Here's how the part is built. I have some questions about the finished solid (model axes, mm). Give positions to 0.01 mm unless a question says otherwise; leave off trailing zeros. Write each loop counter-clockwise with the first axis right and the second up, starting at its lowest first coordinate (ties: lowest second). Pieces come first, ordered by that corner, then holes. Notation, with made-up numbers: (51.25, 29) -> (79.25, 29) arc R24 ccw to (79.25, 41) -> close; hole circle Ø9 at (38.25, 40.25). An arc over 180 degrees is marked (long way). Use one line per item in the form item = value.
```python
from build123d import *

# Parameters (mm, degrees)
TUBE_SQUARE_40_X_40_X_3_2_1_DEPTH = 1920
CUT_EXTRUDE1_DEPTH                = 1921.52076271
SKETCH16_R                        = 2
CUT_EXTRUDE2_DEPTH                = 3


with BuildPart() as part:
    # Sketch15 → Tube (square) 40 X 40 X 3.2(1) (new body)
    with BuildSketch(Plane(origin=(0, 0, 0), x_dir=(-1, 0, 0), z_dir=(0, 1, 0))):
        with BuildLine():
            Line((-13.6, -20), (13.6, -20))
            ThreePointArc((13.6, -20), (18.1254834, -18.1254834), (20, -13.6))
            Line((20, -13.6), (20, 13.6))
            ThreePointArc((20, 13.6), (18.1254834, 18.1254834), (13.6, 20))
            Line((13.6, 20), (-13.6, 20))
            ThreePointArc((-13.6, 20), (-18.1254834, 18.1254834), (-20, 13.6))
            Line((-20, 13.6), (-20, -13.6))
            ThreePointArc((-20, -13.6), (-18.1254834, -18.1254834), (-13.6, -20))
        make_face()
        with BuildLine():
            Line((-13.6, -16.8), (13.6, -16.8))
            ThreePointArc((13.6, -16.8), (15.8627417, -15.8627417), (16.8, -13.6))
            Line((16.8, -13.6), (16.8, 13.6))
            ThreePointArc((16.8, 13.6), (15.8627417, 15.8627417), (13.6, 16.8))
            Line((13.6, 16.8), (-13.6, 16.8))
            ThreePointArc((-13.6, 16.8), (-15.8627417, 15.8627417), (-16.8, 13.6))
            Line((-16.8, 13.6), (-16.8, -13.6))
            ThreePointArc((-16.8, -13.6), (-15.8627417, -15.8627417), (-13.6, -16.8))
        make_face(mode=Mode.SUBTRACT)
    extrude(amount=TUBE_SQUARE_40_X_40_X_3_2_1_DEPTH)

    # Sketch13 → Cut-Extrude1 (cut, through all)
    with BuildSketch(Plane(origin=(0, 0, -20), x_dir=(-1, 0, 0), z_dir=(0, 0, -1))):
        Polygon((20, 1880), (-20, 1920), (20, 1920), align=None)
    extrude(amount=-CUT_EXTRUDE1_DEPTH, mode=Mode.SUBTRACT)

    # Sketch16 → Cut-Extrude2 (cut)
    with BuildSketch(Plane(origin=(20, 0, 0), x_dir=(0, 0, -1), z_dir=(1, 0, 0))):
        with Locations((0, 1900)):
            Circle(SKETCH16_R)
        with Locations((0, 1447)):
            Circle(SKETCH16_R)
        with Locations((0, 1067)):
            Circle(SKETCH16_R)
        with Locations((0, 687)):
            Circle(SKETCH16_R)
    extrude(amount=-CUT_EXTRUDE2_DEPTH, mode=Mode.SUBTRACT)


solid = part.part
```
Q1. I want a section at B-B, the plane y = 239. Write out the boundary of the cut face in (x, z).
Result set:
outline = (-20, -13.6) arc R6.4 ccw to (-13.6, -20) -> (13.6, -20) arc R6.4 ccw to (20, -13.6) -> (20, 13.6) arc R6.4 ccw to (13.6, 20) -> (-13.6, 20) arc R6.4 ccw to (-20, 13.6) -> close; hole (-16.8, -13.6) arc R3.2 ccw to (-13.6, -16.8) -> (13.6, -16.8) arc R3.2 ccw to (16.8, -13.6) -> (16.8, 13.6) arc R3.2 ccw to (13.6, 16.8) -> (-13.6, 16.8) arc R3.2 ccw to (-16.8, 13.6) -> close
Q2. If I drill on line 1 along X through (y, z) = (928, -1); line 2 along X through (y, z) = (1803, 15) (1 decimal), over which ranges is the centre line in solid material (lowest first)? Write a range as from..to.
Result set:
line_1 = -20..-16.8, 16.8..20
line_2 = -19.8..-16.5, 16.5..19.8
Q3. I want a section at A-A, the plane x = -6. Write out the boundary of the cut face in (y, z).
Result set:
outline = (0, -20) -> (1894, -20) -> (1894, -16.8) -> (0, -16.8) -> close; (0, 16.8) -> (1894, 16.8) -> (1894, 20) -> (0, 20) -> close
Q4. Will these pins go through, and if not, where does the flat tip stop? pin 1 Ø1.2 at (y, z) = (687.5, -0.5) entering from +X; pin 2 Ø3 at (y, z) = (1900, 0) entering from -X; pin 3 Ø12 at (x, z) = (8.5, -12.5) entering from -Y.
Result set:
pin_1 = 17
pin_2 = 16.8
pin_3 = 0
